from build123d import *

# Parameters (mm, degrees)
SKETCH_1_W          = 45
SKETCH_1_H          = 45
EXTRUDE_1_DEPTH     = 22.5
EXTRUDE_2_DEPTH     = 24.5
CUT_EXTRUDE_1_DEPTH = 72.48776119
CHAMFER_1_SIZE      = 2
FILLET_1_R          = 3
FILLET_2_R          = 3
SKETCH_5_R          = 12.5
EXTRUDE_3_DEPTH     = 28
SKETCH_6_R          = 4


with BuildPart() as part:
    # ｽｹｯﾁ1 → ﾎﾞｽ - 押し出し1 (new, symmetric)
    with BuildSketch(Plane.XY):
        Rectangle(SKETCH_1_W, SKETCH_1_H)
    extrude(amount=EXTRUDE_1_DEPTH, both=True)

    # ｽｹｯﾁ2 → ﾎﾞｽ - 押し出し2 (add, symmetric)
    with BuildSketch(Plane.XY):
        Polygon((-19.5, -26), (-42.5, -26), (-42.5, -21), (-30.5, -21), (-30.5, 26), (-19.5, 26), align=None)
    extrude_2 = extrude(amount=EXTRUDE_2_DEPTH, both=True)

    # ｽｹｯﾁ3 → ｶｯﾄ - 押し出し1 (cut, symmetric)
    with BuildSketch(Plane.XZ.offset(26)):
        with BuildLine():
            Line((-42.5, -2.75), (-42.5, 2.75))
            Line((-42.5, 2.75), (-37, 2.75))
            ThreePointArc((-37, 2.75), (-34.25, 0), (-37, -2.75))
            Line((-37, -2.75), (-42.5, -2.75))
        make_face()
    cut_extrude_1 = extrude(amount=CUT_EXTRUDE_1_DEPTH, both=True, mode=Mode.SUBTRACT)

    # ｽｹｯﾁ4 → 回転1 (revolve)
    with BuildSketch(Plane.XY, mode=Mode.PRIVATE) as revolve_1_sk:
        Polygon((0, 43.5), (-15, 43.5), (-15, 28.5), (-13, 28.5), (-13, 22.5), (0, 22.5), align=None)
    revolve(revolve_1_sk.sketch.rotate(Axis((0, 0, 0), (0, 1, 0)), 270), axis=Axis((0, 0, 0), (0, 1, 0)))

    # 面取り1
    chamfer_1_edges = [part.edges().sort_by_distance(p)[0] for p in [
        (0, 28.5, 13),
    ]]
    chamfer(chamfer_1_edges, length=CHAMFER_1_SIZE - 0.0001)  # a hair under: the kernel refuses the full size

    # ﾌｨﾚｯﾄ1
    fillet_1_edges = [part.edges().sort_by_distance(p)[0] for p in [
        (0, 43.5, 15),
    ]]
    fillet(fillet_1_edges, radius=FILLET_1_R)

    # ﾐﾗｰ1: ﾎﾞｽ - 押し出し2, ｶｯﾄ - 押し出し1 across plane
    add(extrude_2.mirror(Plane(origin=(0, 0, 0), x_dir=(0, 0, 1), z_dir=(1, 0, 0))))
    add(cut_extrude_1.mirror(Plane(origin=(0, 0, 0), x_dir=(0, 0, 1), z_dir=(1, 0, 0))), mode=Mode.SUBTRACT)

    # ﾌｨﾚｯﾄ2
    fillet_2_edges = [part.edges().sort_by_distance(p)[0] for p in [
        (0, -22.5, -22.5),
        (0, -22.5, 22.5),
        (-25, 26, -24.5),
        (-42.5, -23.5, -24.5),
        (-25, 26, 24.5),
        (-42.5, -23.5, 24.5),
        (0, 22.5, -22.5),
        (0, 22.5, 22.5),
        (42.5, -23.5, 24.5),
        (25, 26, 24.5),
        (25, 26, -24.5),
        (42.5, -23.5, -24.5),
    ]]
    fillet(fillet_2_edges, radius=FILLET_2_R)

    # ｽｹｯﾁ5 → ﾎﾞｽ - 押し出し3 (add)
    with BuildSketch(Plane(origin=(30.5, 0, 0), x_dir=(0, 0, -1), z_dir=(1, 0, 0))):
        with Locations(Location((0, 0, 0), (0, 0, 90))):
            Circle(SKETCH_5_R)
    extrude(amount=EXTRUDE_3_DEPTH)

    # ｽｲｰﾌﾟ1: sweep along a path in ｽｹｯﾁ9
    with BuildLine(Plane.XY) as sweep_1_path:
        Line((58.5, 0), (75, 0))
        ThreePointArc((75, 0), (87.727922061, -5.272077939), (93, -18))
        Line((93, -18), (93, -36))
    # ｽｹｯﾁ6 → ｽｲｰﾌﾟ1 (sweep)
    with BuildSketch(Plane(origin=(58.5, 0, 0), x_dir=(0, 0, -1), z_dir=(1, 0, 0))):
        Circle(SKETCH_6_R)
    sweep(path=sweep_1_path.line)


solid = part.part
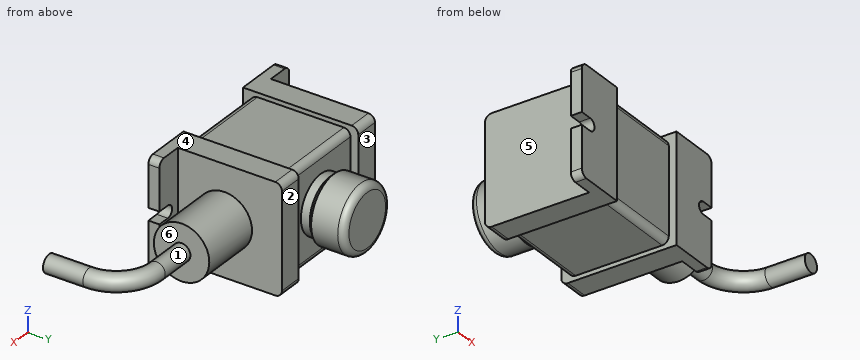
Build history of the part. All positions in model axes, mm. Face numbers are marked on the shaded views. A direction names the side the tool comes from. Give positions to 0.01 mm unless a question says otherwise; leave off trailing zeros. Order: outer loops, then holes, each group sorted by start corner. A loop starts at its lowest first (then second) coordinate and runs counter-clockwise, first axis right, second up. Notation, with made-up numbers: M 68,55.25 L 101,55.25 A9 cw 101,60.25 Z; hole C 15,-28 d6. An arc over 180 degrees is marked long. Put each result on its own line as item: value.
Item 1: Two-plate mould, pull along X, no slides. Class the marked faces 4, 5 and 6: +X half, -X half, draft (parallel to the pull), parting line (faces both ways), or undercut.
From the geometry:
face 4: draft
face 5: -X half
face 6: undercut
Item 2: Probe line 1 (Y direction, x = -15, z = 2); line 2 (X direction, y = 38, z = 0.5). List the from-to ranges inside material, lowest first. Write a range as [from, to].
From the geometry:
line 1: y = [-22.5, 22.5]
line 2: x = [-14.99, 14.99]
Item 3: Slice it at B-B, the plane y = 7.5. Write the cut outline in (x, z).
From the geometry:
outline: M -30.5,-24.5 L -19.5,-24.5 L -19.5,-22.5 L 19.5,-22.5 L 19.5,-24.5 L 30.5,-24.5 L 30.5,-10 L 58.5,-10 L 58.5,10 L 30.5,10 L 30.5,24.5 L 19.5,24.5 L 19.5,22.5 L -19.5,22.5 L -19.5,24.5 L -30.5,24.5 Z
Item 4: Flat gauge pins, fed straight in: pin 1 Ø10 at (x, z) = (73.5, -3.5) entering from +Y; pin 2 Ø11.5 at (x, z) = (-30.5, -6.5) entering from -Y; pin 3 Ø1 at (x, y) = (2.5, -15) entering from -Z; pin 4 Ø12 at (x, y) = (37, 28) entering from -Z. Where does each tip first touch, or does it go through?
From the geometry:
pin 1: stops at y = 4
pin 2: stops at y = -26
pin 3: stops at z = -22.5
pin 4: passes through
Item 5: Slice it at C-C, the plane x = 66.5. Write the cut outline in (y, z).
From the geometry:
outline: C 0,0 d8
Item 6: Slice it at A-A, the plane y = -24.5. Write the cut outline in (x, z).
From the geometry:
outline: M -42.5,-21.5 A3 ccw -39.5,-24.5 L -19.5,-24.5 L -19.5,24.5 L -39.5,24.5 A3 ccw -42.5,21.5 L -42.5,2.75 L -37,2.75 A2.75 cw -37,-2.75 L -42.5,-2.75 Z; M 19.5,-24.5 L 39.5,-24.5 A3 ccw 42.5,-21.5 L 42.5,-2.75 L 37,-2.75 A2.75 cw 37,2.75 L 42.5,2.75 L 42.5,21.5 A3 ccw 39.5,24.5 L 19.5,24.5 Z; C 93,0 d8
Item 7: 3-axis set-ups, long thin cutter, end or side, ignore diameter. For the marked faces 1, 2 and 3: which of +Z, -Z, +X, -X, +Y, -Y reach the whole face in a straight line?
From the geometry:
face 1: none
face 2: +Z, -Z, +X, +Y
face 3: +Z, -Z, -X, +Y
